Autodesk Inventor part; units mm, degrees
ref_plane "YZ Plane" through (0, 0, 0) normal (1, 0, 0) x (0, 1, 0)
ref_plane "XZ Plane" through (0, 0, 0) normal (0, 1, 0) x (-1, 0, 0)
ref_plane "XY Plane" through (0, 0, 0) normal (0, 0, 1) x (1, 0, 0)
sketch "Sketch1" plane through (0, 0, 0) normal (0, 0, 1) x (1, 0, 0)
  circle A0 centre (0, 0) radius 2.6162
  dimension "d0" = 5.2324
extrude "Extrusion1" add sketch "Sketch1" along normal blind 0.508
sketch "Sketch2" plane through (0, 0, 0.508) normal (0, 0, 1) x (1, 0, 0)
  circle A0 centre (0, 0) radius 2.6162
  circle A1 centre (0, 0) radius 2.6162
extrude "Extrusion2" add sketch "Sketch2" along normal blind 2.54 draft -45
sketch "Sketch3" plane through (0, 0, 0) normal (0, 0, -1) x (-1, 0, 0)
  circle A0 centre (0, 0) radius 2.6162
  line L0 (-2.0066, 1.1585) -> (0, 2.317)
  line L1 (0, 2.317) -> (2.0066, 1.1585)
  line L2 (2.0066, 1.1585) -> (2.0066, -1.1585)
  line L3 (2.0066, -1.1585) -> (0, -2.317)
  line L4 (0, -2.317) -> (-2.0066, -1.1585)
  line L5 (-2.0066, -1.1585) -> (-2.0066, 1.1585)
  dimension "d5" = 4.0132
extrude "Extrusion3" add sketch "Sketch3" against normal blind 3.175 contours L0 L1 L2 L3 L4 L5
sketch "Sketch4" plane through (0, 0, 0) normal (0, 0, -1) x (-1, 0, 0)
  circle A0 centre (0, 0) radius 2.6162
  circle A1 centre (0, 0) radius 1.4224
  dimension "d8" = 2.8448
extrude "Extrusion4" cut sketch "Sketch4" against normal through all contours A1
properties part number "MS21042-04"
Input: part model. Units: mm. Frame: model coordinates. A direction names the side the tool comes from. Round coordinates to 2 decimals unless told otherwise and drop trailing zeros. Loops run counter-clockwise (first coordinate to the right, second up) from the corner with the lowest first, then second, coordinate; pieces in that order, holes last. Notation, with made-up numbers: (47.25, 13) -> (93.25, 13) arc R14 cw to (93.25, 25) -> close; hole circle Ø9 at (88.25, 54.25). An arc over 180 degrees is marked (long way). One line per item, written item: value.
(1) Pin query (flat end, axial travel): pin 1 (1.2 mm diameter, centred on y = -0.5, z = 2, fed in from +X); pin 2 (1.9 mm diameter, centred on y = 0, z = 1.5, fed in from -X); pin 3 (1.5 mm diameter, centred on x = -1, z = 2, fed in from +Y); pin 4 (2.5 mm diameter, centred on x = 0, y = 0, fed in from +Z). Return the tip coordinate at first contact, or that it passes through.
Geometry check:
pin 1: x = 2.01
pin 2: x = -2.57
pin 3: y = 2.17
pin 4: through
(2) Section A-A (y = 0). Return the cut outline in (x, z) (3 decimals).
Geometry check:
outline: (-2.616, 0) -> (-1.422, 0) -> (-1.422, 3.175) -> (-2.007, 3.175) -> (-2.007, 1.118) -> (-2.616, 0.508) -> close; (1.422, 0) -> (2.616, 0) -> (2.616, 0.508) -> (2.007, 1.118) -> (2.007, 3.175) -> (1.422, 3.175) -> close
(3) Section C-C (z = 0.4). Return the cut outline in (x, y), plus the area to 3 significant figures.
Geometry check:
outline: circle Ø5.23 at (0, 0); hole circle Ø2.84 at (0, 0)
area: 15.1 mm2
(4) Mould query, pull axis Y, two halves, no side actions, for faces 4 (the face through (-1.02, -1.73, 1.97)), 5 (the face through (0.31, -1.39, 1.57)), 6 (the face through (-2.007, 0, 2)), 7 (the face through (-0.989, 1.746, 1.975)). Classes: pulls with the +Y half, pulls with the -Y half, needs draft (parallel to the pull), parting line crosses it, or undercut.
Geometry check:
face 4: pulls with the -Y half
face 5: undercut
face 6: needs draft
face 7: pulls with the +Y half
(5) Set-up query: faces 1 (the face through (0.989, -1.746, 1.975)), 2 (the face through (1.02, 1.73, 1.97)), 3 (the face through (-0.567, 2.554, 0.25)). Return all of +Z, -Z, +X, -X, +Y, -Y with unobstructed straight access to the full face (end or side cutting, diameter ignored); none if empty.
Geometry check:
face 1: +Z, +X, -Y
face 2: +Z, +X, +Y
face 3: +Z, -Z
(6) Material intervals for line 1 (X direction, y = -0.5, z = 1.8); line 2 (Y direction, x = -0.3, z = 2.5); line 3 (X direction, y = -0.8, z = 3), sorted ascending. Write a range as [from, to].
Geometry check:
line 1: [-2.01, -1.33], [1.33, 2.01]
line 2: [-2.14, -1.39], [1.39, 2.14]
line 3: [-2.01, -1.18], [1.18, 2.01]
(7) Section B-B (z = 2.5). Return the cut outline in (x, y), plus the area to 3 significant figures.
Geometry check:
outline: (-2.01, -1.16) -> (0, -2.32) -> (2.01, -1.16) -> (2.01, 1.16) -> (0, 2.32) -> (-2.01, 1.16) -> close; hole circle Ø2.84 at (0, 0)
area: 7.59 mm2
